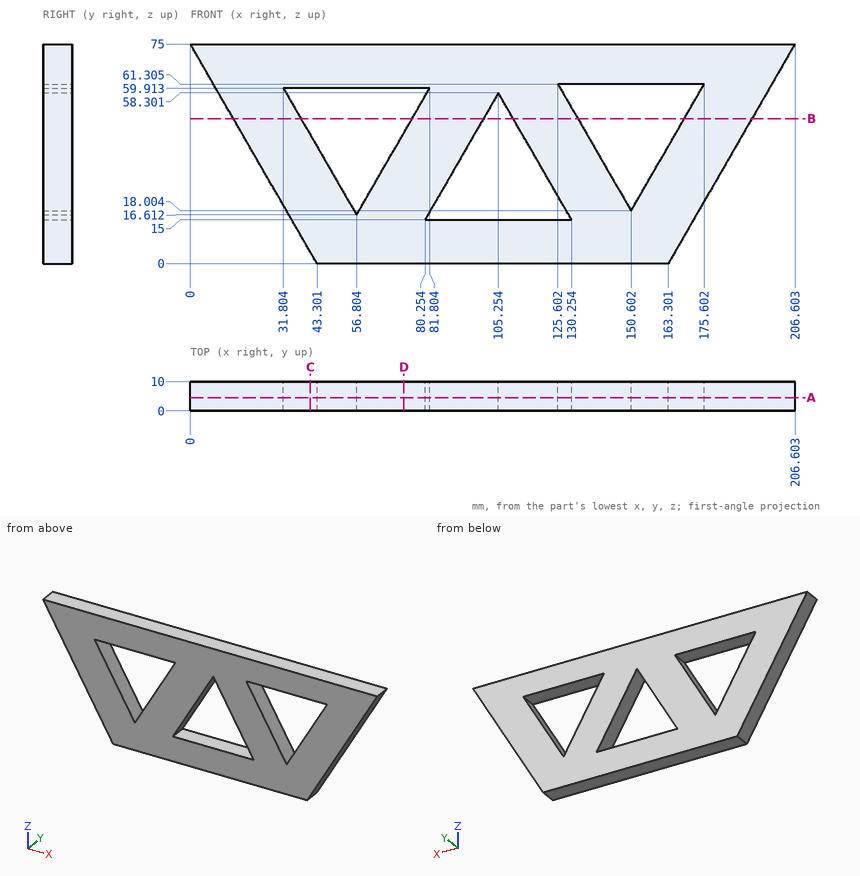
The drawing under review shows one solid part. Ordinate dimensions are in mm from its lowest x, y, z. Coordinates: 2 decimals unless noted, no trailing zeros. Order: outer loops, then holes, each group sorted by start corner. A loop starts at its lowest first (then second) coordinate and runs counter-clockwise, first axis right, second up. Notation, with made-up numbers: (-27.5, 84.5) -> (-14.5, 84.5) arc R17 cw to (-14.5, 100.5) -> close; hole circle Ø9 at (37.5, 79). An arc over 180 degrees is marked (long way). Return JSON: item names as keys, results as strings.
1. For line 1 (X direction, y = 6, z = 44) (1 decimal); line 2 (X direction, y = 5.5, z = 48.5) (1 decimal); line 3 (Z direction, x = 76, y = 6.25) (1 decimal), list the stretches that pass through material, from the lowest coordinate up. Write a range as from..to.
Answer block:
{"line 1": "17.9..41, 72.6..97, 113.5..135.6, 165.6..188.7", "line 2": "15.3..38.4, 75.2..99.6, 110.9..133, 168.2..191.3", "line 3": "0..49.9, 59.9..75"}
2. We need section D-D on x = 73. Write out the cut boundary in (y, z).
Answer block:
{"outline": "(0, 0) -> (10, 0) -> (10, 44.66) -> (0, 44.66) -> close; (0, 59.91) -> (10, 59.91) -> (10, 75) -> (0, 75) -> close"}
3. We need section C-C on x = 41. Write out the cut boundary in (y, z) (1 decimal), and give its area (3 significant figures).
Answer block:
{"outline": "(0, 4) -> (10, 4) -> (10, 44) -> (0, 44) -> close; (0, 59.9) -> (10, 59.9) -> (10, 75) -> (0, 75) -> close", "area": "551 mm²"}
4. For pin 1 Ø2 at (x, z) = (111.5, 11.5) entering from -Y; pin 2 Ø4 at (y, z) = (6.5, 38.5) entering from +X (1 decimal), all flat-tipped, find the tip position at first contact; note any pin that passes through.
Answer block:
{"pin 1": "y = 0", "pin 2": "x = 186.7"}
5. We need section A-A on y = 4.5. Write out the cut boundary in (x, z) (1 decimal).
Answer block:
{"outline": "(0, 75) -> (43.3, 0) -> (163.3, 0) -> (206.6, 75) -> close; hole (31.8, 59.9) -> (56.8, 16.6) -> (81.8, 59.9) -> close; hole (80.3, 15) -> (130.3, 15) -> (105.3, 58.3) -> close; hole (125.6, 61.3) -> (150.6, 18) -> (175.6, 61.3) -> close"}
6. We need section B-B on z = 49.5. Write out the cut boundary in (x, y) (1 decimal).
Answer block:
{"outline": "(14.7, 0) -> (37.8, 0) -> (37.8, 10) -> (14.7, 10) -> close; (75.8, 0) -> (100.2, 0) -> (100.2, 10) -> (75.8, 10) -> close; (110.3, 0) -> (132.4, 0) -> (132.4, 10) -> (110.3, 10) -> close; (168.8, 0) -> (191.9, 0) -> (191.9, 10) -> (168.8, 10) -> close"}
